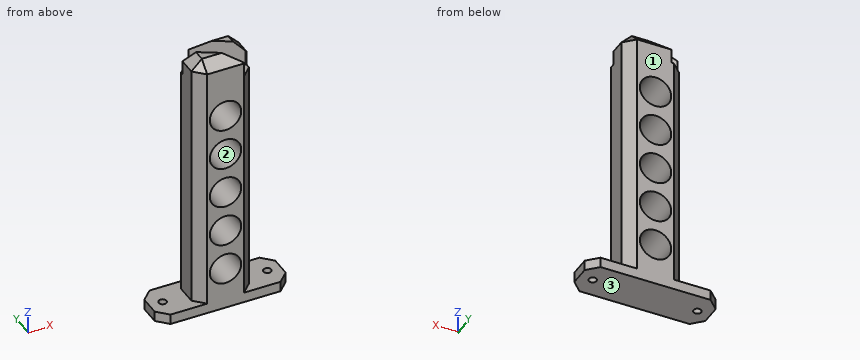
from build123d import *

# Parameters (mm, degrees)
F0_W     = 63.5
F0_H     = 20
F0_R     = 1.875
F1_DEPTH = 5
F2_W     = 27.94
F2_H     = 20
F3_DEPTH = 127
F4_R     = 7.62
F5_DEPTH = 25.4
F6_SIZE  = 5.08
F8_DEPTH = 12


with BuildPart() as f1:
    # F0 (on Top) → F1 (new body)
    with BuildSketch(Plane.XY):
        Rectangle(F0_W, F0_H)
        with Locations((-25.4, 0)):
            Circle(F0_R, mode=Mode.SUBTRACT)
        with Locations((25.4, 0)):
            Circle(F0_R, mode=Mode.SUBTRACT)
    extrude(amount=F1_DEPTH)

    # F2 (on face) → F3 (join)
    with BuildSketch(Plane.XY.offset(5)):
        Rectangle(F2_W, F2_H)
    extrude(amount=F3_DEPTH)

    # F4 (on face) → F5 (cut)
    with BuildSketch(Plane.XZ.offset(10)):
        with Locations((0, 102.0142971116)):
            Circle(F4_R)
        with Locations((0, 81.6942971116)):
            Circle(F4_R)
        with Locations((0, 61.3742971116)):
            Circle(F4_R)
        with Locations((0, 41.0542971116)):
            Circle(F4_R)
        with Locations((0, 20.7342971116)):
            Circle(F4_R)
    extrude(amount=-F5_DEPTH, mode=Mode.SUBTRACT)

    # F6
    f6_edges = [f1.edges().sort_by_distance(p)[0] for p in [
        (-13.97, -10, 68.5),
        (13.97, -10, 68.5),
        (13.97, 10, 68.5),
        (-13.97, 10, 68.5),
        (-13.97, 0, 132),
        (0, -10, 132),
        (13.97, 0, 132),
        (0, 10, 132),
        (-31.75, -10, 2.5),
        (31.75, 10, 2.5),
        (31.75, -10, 2.5),
        (-31.75, 10, 2.5),
    ]]
    chamfer(f6_edges, length=F6_SIZE)

    # F7 (on face) → F8 (cut)
    with BuildSketch(Plane.XY.offset(132)):
        with BuildLine():
            ThreePointArc((9.1241109486, -9.7629955106), (15.03217082, -8.1799356392), (13.4491109486, -2.2718757679))
            Line((13.4491109486, -2.2718757679), (-10.0027512471, 11.2680631838))
            ThreePointArc((-10.0027512471, 11.2680631838), (-15.9108111184, 9.6850033125), (-14.3277512471, 3.7769434411))
            Line((-14.3277512471, 3.7769434411), (9.1241109486, -9.7629955106))
        make_face()
    extrude(amount=-F8_DEPTH, mode=Mode.SUBTRACT)


solid = f1.part
Model file for the job. Use its own axes, mm. Face numbers are marked on the shaded views. Coordinates: 2 decimals unless noted, no trailing zeros. Write each loop counter-clockwise with the first axis right and the second up, starting at its lowest first coordinate (ties: lowest second). Pieces come first, ordered by that corner, then holes. Notation, with made-up numbers: (-22, -29.75) - (-18, -29.75) arc R24 cw to (-18, 2.25) - close; hole circle Ø2 at (42.25, -27.5). An arc over 180 degrees is marked (long way). Write each question's results on one line, items separated by ' | '. Start each with the question number.
1) Cut at C-C (z = 30.5). Write the cut outline in (x, y).
2) Cut at B-B (z = 57). Write the cut outline in (x, y).
3) Flat gauge pins, fed straight in: P1, Ø4.5, axis at x = 25.4, y = 0, coming from the +Z side; P2, Ø20, axis at x = 0, z = 20.73, coming from the -Y side; P3, Ø8, axis at y = 1.5, z = 41, coming from the +X side; P4, Ø3, axis at y = -1, z = 82.5, coming from the -X side. Where does each tip first touch, or does it go through?
4) Cut at A-A (x = -25.4). Write the cut outline in (y, z) (3 decimals), then the cut area to 4 significant figures.
5) Probe line 1 along Z through (x, y) = (0, 4.75); line 2 along X through (y, z) = (-3, 82); line 3 along Z through (x, y) = (1, -3). List the from-to ranges inside material, lowest first. Write a range as from..to.
6) Mould opens along Z. For the marked faces 1, 2 and 3 say: pulls with the +Z half, pulls with the -Z half, needs draft (parallel to the pull), parting line crosses it, or undercut.
7) Cut at D-D (y = 6.75). Write the cut outline in (x, z).
Returned:
1) outline: (-13.97, -4.92) - (-8.89, -10) - (8.89, -10) - (13.97, -4.92) - (13.97, 4.92) - (8.89, 10) - (-8.89, 10) - (-13.97, 4.92) - close
2) outline: (-13.97, -4.92) - (-8.89, -10) - (-6.24, -10) - (-6.24, 10) - (-8.89, 10) - (-13.97, 4.92) - close; (6.24, -10) - (8.89, -10) - (13.97, -4.92) - (13.97, 4.92) - (8.89, 10) - (6.24, 10) - close
3) P1: z = 5 | P2: y = -10 | P3: x = 13.97 | P4: x = -13.97
4) outline: (-10, 0) - (-1.875, 0) - (-1.875, 5) - (-10, 5) - close; (1.875, 0) - (10, 0) - (10, 5) - (1.875, 5) - close | area: 81.25 mm^2
5) line 1: 0..13.11, 28.35..33.43, 48.67..53.75, 68.99..74.07, 89.31..94.39, 109.63..120 | line 2: -13.97..-7.61, 7.61..13.97 | line 3: 0..13.18, 28.29..33.5, 48.61..53.82, 68.93..74.14, 89.25..94.46, 109.57..120
6) face 1: needs draft | face 2: undercut | face 3: pulls with the -Z half
7) outline: (-29.92, 0) - (29.92, 0) - (29.92, 5) - (12.14, 5) - (12.14, 126.92) - (8.89, 130.17) - (-2.18, 130.17) - (-2.18, 120) - (-12.14, 120) - (-12.14, 5) - (-29.92, 5) - close; hole circle Ø15.24 at (0, 20.73); hole circle Ø15.24 at (0, 41.05); hole circle Ø15.24 at (0, 61.37); hole circle Ø15.24 at (0, 81.69); hole circle Ø15.24 at (0, 102.01)
